from build123d import *

# Parameters (mm, degrees)
AUFSATZ_LINEAR_AUSTRAGEN2_DEPTH = 7
VERRUNDUNG2_R                   = 1


with BuildPart() as part:
    # Skizze1 → Rotation1 (revolve)
    with BuildSketch(Plane(origin=(0, 0, 0), x_dir=(1, 0, 0), z_dir=(0, 1, 0))):
        with BuildLine():
            Line((-7, 0), (-7, 2.8))
            Line((-7, 2.8), (-15, 6))
            ThreePointArc((-15, 6), (-16.486832981, 3.16227766), (-17, 0))
            Line((-17, 0), (-7, 0))
        make_face()
    revolve(axis=Axis((-7.719127457, 0, 0), (-1, 0, 0)))

    # Skizze1_3 → Aufsatz-Linear austragen2 (add, symmetric)
    with BuildSketch(Plane(origin=(0, 0, 0), x_dir=(1, 0, 0), z_dir=(0, 1, 0))):
        Polygon((-7, -7), (7, -7), (7, 0), (7, 7), (-7, 7), (-7, 0), align=None)
    extrude(amount=AUFSATZ_LINEAR_AUSTRAGEN2_DEPTH, both=True)

    # Verrundung2
    verrundung2_edges = [part.edges().sort_by_distance(p)[0] for p in [
        (0, -7, 7),
        (-7, 0, 7),
        (7, -7, 0),
        (7, 0, 7),
        (0, 7, -7),
        (7, 0, -7),
        (-7, 7, 0),
        (-7, 0, -7),
        (0, 7, 7),
        (7, 7, 0),
        (-7, -7, 0),
        (0, -7, -7),
    ]]
    fillet(verrundung2_edges, radius=VERRUNDUNG2_R)


solid = part.part
Build history of the part. All positions in model axes, mm. A direction names the side the tool comes from. Round coordinates to 2 decimals unless told otherwise and drop trailing zeros. Write each loop counter-clockwise with the first axis right and the second up, starting at its lowest first coordinate (ties: lowest second). Pieces come first, ordered by that corner, then holes. Notation, with made-up numbers: M 64,46.25 L 81,46.25 A7 cw 81,56.25 Z; hole C 42,81.25 d2. An arc over 180 degrees is marked long. Use CSV: the item, a comma, the result in double quotes.
1. Flat gauge pins, fed straight in: pin 1 (1 mm diameter, centred on x = -8, y = 0.5, fed in from -Z); pin 2 (6 mm diameter, centred on x = -14.5, y = 4.5, fed in from +Z); pin 3 (8 mm diameter, centred on x = -9, y = -5.5, fed in from -Z); pin 4 (4 mm diameter, centred on y = -3, z = -2, fed in from -X). Where does each tip first touch, or does it go through?
Reply:
pin 1,"stops at z = -3.37"
pin 2,"stops at z = 5.8"
pin 3,"stops at z = -7"
pin 4,"stops at x = -16.87"
2. Two-plate mould, pull along X, no slides. Class faces 3 (the face through (6.715, 0.084, -6.699)), 4 (the face through (-9.278, 3.623, 0.805)), 5 (the face through (-0.084, 6.715, -6.699)): +X half, -X half, draft (parallel to the pull), parting line (faces both ways), or undercut.
Reply:
face 3,"+X half"
face 4,"undercut"
face 5,"draft"
3. Saw through at D-D (x = -8.25). Give the cut face in (y, z), plus the area to 3 significant figures.
Reply:
outline,"C 0,0 d6.6"
area,"34.2 mm²"
4. Tool access for faces 1 (the face through (-7, 1, 3)), 2 (the face through (0.084, -6.699, 6.715)): list every direction of +Z, -Z, +X, -X, +Y, -Y with a clear straight run to the whole face (end or side of a thin tool).
Reply:
face 1,"none"
face 2,"+Z, +X, -X, -Y"
5. Saw through at A-A (y = 0). Give the cut face in (x, z), plus the area to 3 significant figures.
Reply:
outline,"M -15,-6 L -7,-2.8 L -7,-6 A1 ccw -6,-7 L 6,-7 A1 ccw 7,-6 L 7,6 A1 ccw 6,7 L -6,7 A1 ccw -7,6 L -7,2.8 L -15,6 A10 ccw Z"
area,"282 mm²"
6. Wall check: probe 1 along X at (y, z) = (2.5, -6); probe 2 along X at (y, z) = (-1.5, 3); probe 3 along X at (y, z) = (-1.75, -2.75). Give the ranges that are in metal, low to high. Write a range as from..to.
Reply:
probe 1,"x = -7..7"
probe 2,"x = -16.42..-8.39, -7..7"
probe 3,"x = -16.45..-8.15, -7..7"
7. Saw through at C-C (x = -14). Give the cut face in (y, z).
Reply:
outline,"C 0,0 d11.2"
